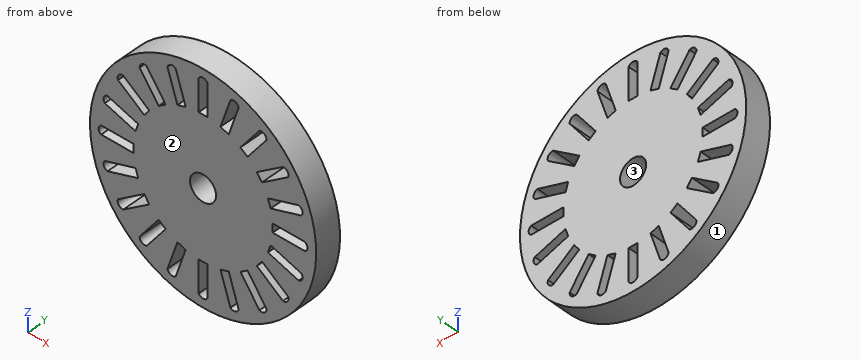
```python
from build123d import *

# Parameters (mm, degrees)
CROQUIS1_R              = 13
CROQUIS1_R_2            = 1.5
SALIENTE_EXTRUIR1_DEPTH = 3
CORTAR_EXTRUIR1_DEPTH   = 3
MATRIZC1_COUNT          = 20


with BuildPart() as part:
    # Croquis1 → Saliente-Extruir1 (new body)
    with BuildSketch(Plane(origin=(0, 0, 0), x_dir=(1, 0, 0), z_dir=(0, 1, 0))):
        with Locations(Location((0, 0, 0), (0, 0, 270))):
            Circle(CROQUIS1_R)
        with Locations(Location((0, 0, 0), (0, 0, 270))):
            Circle(CROQUIS1_R_2, mode=Mode.SUBTRACT)
    extrude(amount=SALIENTE_EXTRUIR1_DEPTH)

    # Croquis2 → Cortar-Extruir1 (cut)
    with BuildSketch(Plane(origin=(0, 3, 0), x_dir=(1, 0, 0), z_dir=(0, 1, 0))):
        with BuildLine():
            Line((-0.5, 8), (0.5, 8))
            Line((0.5, 8), (0.5, 11.712659584))
            ThreePointArc((0.5, 11.712659584), (0.000139252, 12), (-0.5, 11.713144616))
            Line((-0.5, 11.713144616), (-0.5, 8))
        make_face()
    cortar_extruir1 = extrude(amount=-CORTAR_EXTRUIR1_DEPTH, mode=Mode.SUBTRACT)

    # MatrizC1: Cortar-Extruir1 ×20 about axis
    matrizc1_axis = Axis((0, 0, 0), (0, 1, 0))
    for i in range(1, MATRIZC1_COUNT):
        add(cortar_extruir1.rotate(matrizc1_axis, i * 360 / MATRIZC1_COUNT), mode=Mode.SUBTRACT)


solid = part.part
```
Model file for the job. Use its own axes, mm. Face numbers are marked on the shaded views. Give positions to 0.01 mm unless a question says otherwise; leave off trailing zeros. Loops run counter-clockwise (first coordinate to the right, second up) from the corner with the lowest first, then second, coordinate; pieces in that order, holes last. Notation, with made-up numbers: (21.25, 73.5) -> (53.25, 73.5) arc R18 cw to (53.25, 85.5) -> close; hole circle Ø5 at (-29, -0.5). An arc over 180 degrees is marked (long way). Use CSV: the item, a comma, the result in double quotes. Start each with the question number.
1) Mould opens along Z. For the marked faces 1, 2 and 3 say: released by +Z, released by -Z, zero draft, split by the parting line, or undercut.
2) Flat gauge pins, fed straight in: pin 1 Ø0.9 at (y, z) = (1, 9) entering from -X; pin 2 Ø0.9 at (x, y) = (-10.5, 2) entering from +Z; pin 3 Ø1.5 at (x, y) = (-9, 1) entering from +Z. Where does each tip first touch, or does it go through?
3) Slice it at C-C on y = 0.45. Give the number of separate pieces and of enclosed holes in the cut face, plus the area to 3 significant figures.
4) Wall check: line 1 (X direction, y = 1.7, z = 0); line 2 (Z direction, x = -6.5, y = 1.9); line 3 (X direction, y = 1.9, z = 9.75). Give the ranges that are in metal, low to high.
5) Slice it at A-A on z = 0. Give the cut face in (x, y).
6) Slice it at B-B on x = 0. Give the cut face in (y, z), plus the area to 3 significant figures.
Computed values:
1,face 1,"split by the parting line"
1,face 2,"zero draft"
1,face 3,"undercut"
2,pin 1,"stops at x = -9.79"
2,pin 2,"stops at z = 8.25"
2,pin 3,"stops at z = 10.05"
3,separate pieces,"1"
3,enclosed holes,"21"
3,area,"446 mm^2"
4,line 1,"x = -13 to -12, -8 to -1.5, 1.5 to 8, 12 to 13"
4,line 2,"z = -11.26 to -9.78, -8.1 to -5.34, -4.66 to 4.66, 5.34 to 8.1, 9.78 to 11.26"
4,line 3,"x = -8.6 to -6.99, -6.47 to -3.69, -2.64 to -0.5, 0.5 to 2.64, 3.69 to 6.47, 6.99 to 8.6"
5,outline,"(-13, 0) -> (-12, 0) -> (-12, 3) -> (-13, 3) -> close; (-8, 0) -> (-1.5, 0) -> (-1.5, 3) -> (-8, 3) -> close; (1.5, 0) -> (8, 0) -> (8, 3) -> (1.5, 3) -> close; (12, 0) -> (13, 0) -> (13, 3) -> (12, 3) -> close"
6,outline,"(0, -13) -> (3, -13) -> (3, -12) -> (0, -12) -> close; (0, -8) -> (3, -8) -> (3, -1.5) -> (0, -1.5) -> close; (0, 1.5) -> (3, 1.5) -> (3, 8) -> (0, 8) -> close; (0, 12) -> (3, 12) -> (3, 13) -> (0, 13) -> close"
6,area,"45.0 mm^2"
